Geometry: final body of the model. Coordinates: model frame, mm. Face numbers are marked on the shaded views. A direction names the side the tool comes from. Give positions to 0.01 mm unless a question says otherwise; leave off trailing zeros. Write each loop counter-clockwise with the first axis right and the second up, starting at its lowest first coordinate (ties: lowest second). Pieces come first, ordered by that corner, then holes. Notation, with made-up numbers: (-14.5, 12.25) -> (37.5, 12.25) arc R14 ccw to (37.5, 28.25) -> close; hole circle Ø2 at (-12.75, 8.5). An arc over 180 degrees is marked (long way). Answer in a Markdown table with one row per item. Add a question column.
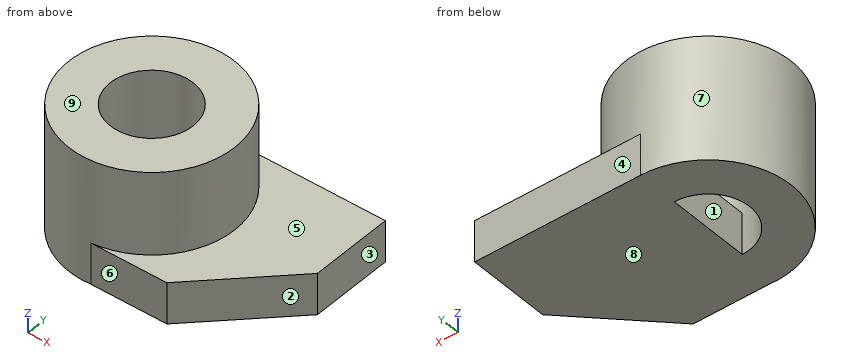
from build123d import *

# Parameters (mm, degrees)
F0_R     = 12.7
F0_R_2   = 6.35
F1_DEPTH = 19.05
F3_DEPTH = 6.35


with BuildPart() as f1:
    # F0 (on Top) → F1 (new body)
    with BuildSketch(Plane.XY):
        Circle(F0_R)
        Circle(F0_R_2, mode=Mode.SUBTRACT)
    extrude(amount=F1_DEPTH)

    # F2 (on Top) → F3 (join)
    with BuildSketch(Plane.XY):
        Polygon((25.4, 12.7), (0, 12.7), (0, -12.655177), (12.7, -12.655177), (25.4, 0), align=None)
    extrude(amount=F3_DEPTH)


solid = f1.part
Q1. Access query for the marked faces 5, 6, 7, 8 and 9. Directions: +Z, -Z, +X, -X, +Y, -Y. A direction counts if a zero-diameter tool reaches every point of the face in a straight line with its end or side. Return the directions, or none.
Q2. Section B-B on z = 7.5. Return loops of the section in (x, y).
Q3. Section C-C on x = 4.5. Return loops of the section in (y, z), and give its area (3 significant figures).
Q4. Contact query for flat-ended pins moving along their axis: pin 1 Ø10 at (y, z) = (-9.5, 16) entering from +X; pin 2 Ø4 at (x, z) = (-7, 9) entering from +Y; pin 3 Ø6 at (x, z) = (15.5, 6.5) entering from +Y; pin 4 Ø10 at (x, z) = (9.5, 16) entering from +Y. Output: stop coordinate, or through.
Q5. Pull-direction query (Y, two-part tool) for the marked faces 1, 2, 3 and 4; classes: +Y half, -Y half, draft (parallel to the pull), parting line (faces both ways), or undercut.
Q6. Section D-D on y = 9.75. Return loops of the section in (x, z).
Q7. Line query: probe 1 along X at (y, z) = (0, 11.5); probe 2 along Y at (x, z) = (5.5, 4.75). Output: solid intervals per line, ascending. Write a range as from..to.
Q8. Section A-A on y = 2.25. Return loops of the section in (x, z).
Checks:
| question | item | result |
|---|---|---|
| 1 | face 5 | +Z, +X |
| 1 | face 6 | +Z, -Z, +X, -Y |
| 1 | face 7 | +Z |
| 1 | face 8 | -Z, +X, -X, +Y, -Y |
| 1 | face 9 | +Z, +X, -X, +Y, -Y |
| 2 | outline | circle Ø25.4 at (0, 0); hole circle Ø12.7 at (0, 0) |
| 3 | outline | (-12.66, 0) -> (12.7, 0) -> (12.7, 6.35) -> (11.88, 6.35) -> (11.88, 19.05) -> (4.48, 19.05) -> (4.48, 6.35) -> (-4.48, 6.35) -> (-4.48, 19.05) -> (-11.88, 19.05) -> (-11.88, 6.35) -> (-12.66, 6.35) -> close |
| 3 | area | 349 mm^2 |
| 4 | pin 1 | x = 11.88 |
| 4 | pin 2 | y = 11.67 |
| 4 | pin 3 | y = 12.7 |
| 4 | pin 4 | y = 11.88 |
| 5 | face 1 | undercut |
| 5 | face 2 | -Y half |
| 5 | face 3 | draft |
| 5 | face 4 | +Y half |
| 6 | outline | (-8.14, 0) -> (25.4, 0) -> (25.4, 6.35) -> (8.14, 6.35) -> (8.14, 19.05) -> (-8.14, 19.05) -> close |
| 7 | probe 1 | -12.7..-6.35, 6.35..12.7 |
| 7 | probe 2 | -12.66..12.7 |
| 8 | outline | (-12.5, 0) -> (-5.94, 0) -> (-5.94, 19.05) -> (-12.5, 19.05) -> close; (0, 0) -> (25.4, 0) -> (25.4, 6.35) -> (12.5, 6.35) -> (12.5, 19.05) -> (5.94, 19.05) -> (5.94, 6.35) -> (0, 6.35) -> close |
